```python
from build123d import *

# Parameters (mm, degrees)
IZIM1_R                     = 16
Y_KSEKLIK_EKSTR_ZYON1_DEPTH = 5
IZIM2_R                     = 8
Y_KSEKLIK_EKSTR_ZYON2_DEPTH = 19.7
KES_EKSTR_ZYON1_REACH       = 35.498
IZIM3_R                     = 4
KES_EKSTR_ZYON2_REACH       = 35.498
IZIM4_R                     = 1.75
IZIM4_3_R                   = 3.25
IZIM4_3_R_2                 = 1.75
KES_EKSTR_ZYON3_DEPTH       = 3.7
IZIM5_R                     = 6.5
KES_EKSTR_ZYON4_DEPTH       = 1.3
KES_EKSTR_ZYON5_START       = -23.4
IZIM5_2_R                   = 6.5
KES_EKSTR_ZYON5_DEPTH       = 1.3
KES_EKSTR_ZYON7_START       = -0.3
IZIM7_R                     = 9.5
IZIM7_R_2                   = 8
KES_EKSTR_ZYON7_DEPTH       = 0.3
IZIM8_R                     = 8
IZIM8_R_2                   = 7.5
KES_EKSTR_ZYON8_DEPTH       = 1
PAH1_SIZE                   = 0.5
Y_KSEKLIK_EKSTR_ZYON3_START = 0.5
IZIM9_R                     = 4.5
IZIM9_R_2                   = 4
Y_KSEKLIK_EKSTR_ZYON3_DEPTH = 0.5
Y_KSEKLIK_EKSTR_ZYON4_START = -22.1
IZIM9_2_R                   = 4.5
IZIM9_2_R_2                 = 4
Y_KSEKLIK_EKSTR_ZYON4_DEPTH = 0.5
PAH2_SIZE                   = 0.5


with BuildPart() as part:
    # Çizim1 → Yükseklik-Ekstrüzyon1 (new body)
    with BuildSketch(Plane.XY):
        Circle(IZIM1_R)
    extrude(amount=Y_KSEKLIK_EKSTR_ZYON1_DEPTH)

    # Çizim2 → Yükseklik-Ekstrüzyon2 (add)
    with BuildSketch(Plane.XY.offset(5)):
        Circle(IZIM2_R)
    extrude(amount=Y_KSEKLIK_EKSTR_ZYON2_DEPTH)

    # Çizim3 → Kes-Ekstrüzyon1 (cut, up to next)
    with BuildSketch(Plane.XY.offset(24.7), mode=Mode.PRIVATE) as kes_ekstr_zyon1_sk1:
        Circle(IZIM3_R)
    kes_ekstr_zyon1_tool1 = extrude(kes_ekstr_zyon1_sk1.sketch, amount=-KES_EKSTR_ZYON1_REACH, mode=Mode.PRIVATE) & part.part
    add(kes_ekstr_zyon1_tool1.solids().sort_by_distance((0, 0, 24.7))[0], mode=Mode.SUBTRACT)

    # Çizim4 → Kes-Ekstrüzyon2 (cut, up to next)
    with BuildSketch(Plane(origin=(0, 0, 0), x_dir=(-1, 0, 0), z_dir=(0, 0, -1)), mode=Mode.PRIVATE) as kes_ekstr_zyon2_sk1:
        with Locations((0, 12)):
            Circle(IZIM4_R)
    kes_ekstr_zyon2_tool1 = extrude(kes_ekstr_zyon2_sk1.sketch, amount=-KES_EKSTR_ZYON2_REACH, mode=Mode.PRIVATE) & part.part
    # Çizim4 → Kes-Ekstrüzyon2 (cut, up to next)
    with BuildSketch(Plane(origin=(0, 0, 0), x_dir=(-1, 0, 0), z_dir=(0, 0, -1)), mode=Mode.PRIVATE) as kes_ekstr_zyon2_sk2:
        with Locations((12, 0)):
            Circle(IZIM4_R)
    kes_ekstr_zyon2_tool2 = extrude(kes_ekstr_zyon2_sk2.sketch, amount=-KES_EKSTR_ZYON2_REACH, mode=Mode.PRIVATE) & part.part
    # Çizim4 → Kes-Ekstrüzyon2 (cut, up to next)
    with BuildSketch(Plane(origin=(0, 0, 0), x_dir=(-1, 0, 0), z_dir=(0, 0, -1)), mode=Mode.PRIVATE) as kes_ekstr_zyon2_sk3:
        with Locations((0, -12)):
            Circle(IZIM4_R)
    kes_ekstr_zyon2_tool3 = extrude(kes_ekstr_zyon2_sk3.sketch, amount=-KES_EKSTR_ZYON2_REACH, mode=Mode.PRIVATE) & part.part
    # Çizim4 → Kes-Ekstrüzyon2 (cut, up to next)
    with BuildSketch(Plane(origin=(0, 0, 0), x_dir=(-1, 0, 0), z_dir=(0, 0, -1)), mode=Mode.PRIVATE) as kes_ekstr_zyon2_sk4:
        with Locations((-12, 0)):
            Circle(IZIM4_R)
    kes_ekstr_zyon2_tool4 = extrude(kes_ekstr_zyon2_sk4.sketch, amount=-KES_EKSTR_ZYON2_REACH, mode=Mode.PRIVATE) & part.part
    add(kes_ekstr_zyon2_tool1.solids().sort_by_distance((0, 12, 0))[0], mode=Mode.SUBTRACT)
    add(kes_ekstr_zyon2_tool2.solids().sort_by_distance((-12, 0, 0))[0], mode=Mode.SUBTRACT)
    add(kes_ekstr_zyon2_tool3.solids().sort_by_distance((0, -12, 0))[0], mode=Mode.SUBTRACT)
    add(kes_ekstr_zyon2_tool4.solids().sort_by_distance((12, 0, 0))[0], mode=Mode.SUBTRACT)

    # Çizim4<3> → Kes-Ekstrüzyon3 (cut)
    # profile 1 of 4: a face of its own
    with BuildSketch(Plane(origin=(0, 0, 0), x_dir=(-1, 0, 0), z_dir=(0, 0, -1))):
        with Locations((0, 12)):
            Circle(IZIM4_3_R)
        with Locations((0, 12)):
            Circle(IZIM4_3_R_2, mode=Mode.SUBTRACT)
    # profile 2 of 4: a face of its own
    with BuildSketch(Plane(origin=(0, 0, 0), x_dir=(-1, 0, 0), z_dir=(0, 0, -1))):
        with Locations((12, 0)):
            Circle(IZIM4_3_R)
        with Locations((12, 0)):
            Circle(IZIM4_3_R_2, mode=Mode.SUBTRACT)
    # profile 3 of 4: a face of its own
    with BuildSketch(Plane(origin=(0, 0, 0), x_dir=(-1, 0, 0), z_dir=(0, 0, -1))):
        with Locations((0, -12)):
            Circle(IZIM4_3_R)
        with Locations((0, -12)):
            Circle(IZIM4_3_R_2, mode=Mode.SUBTRACT)
    # profile 4 of 4: a face of its own
    with BuildSketch(Plane(origin=(0, 0, 0), x_dir=(-1, 0, 0), z_dir=(0, 0, -1))):
        with Locations((-12, 0)):
            Circle(IZIM4_3_R)
        with Locations((-12, 0)):
            Circle(IZIM4_3_R_2, mode=Mode.SUBTRACT)
    extrude(amount=-KES_EKSTR_ZYON3_DEPTH, mode=Mode.SUBTRACT)

    # Çizim5 → Kes-Ekstrüzyon4 (cut)
    with BuildSketch(Plane.XY.offset(24.7)):
        Circle(IZIM5_R)
    extrude(amount=-KES_EKSTR_ZYON4_DEPTH, mode=Mode.SUBTRACT)

    # Çizim5<2> → Kes-Ekstrüzyon5 (cut)
    with BuildSketch(Plane.XY.offset(24.7).offset(KES_EKSTR_ZYON5_START)):
        Circle(IZIM5_2_R)
    extrude(amount=-KES_EKSTR_ZYON5_DEPTH, mode=Mode.SUBTRACT)

    # Çizim7 → Kes-Ekstrüzyon7 (cut)
    with BuildSketch(Plane.XY.offset(5).offset(KES_EKSTR_ZYON7_START)):
        Circle(IZIM7_R)
        Circle(IZIM7_R_2, mode=Mode.SUBTRACT)
    extrude(amount=KES_EKSTR_ZYON7_DEPTH, mode=Mode.SUBTRACT)

    # Çizim8 → Kes-Ekstrüzyon8 (cut)
    with BuildSketch(Plane.XY.offset(4.7)):
        Circle(IZIM8_R)
        Circle(IZIM8_R_2, mode=Mode.SUBTRACT)
    extrude(amount=KES_EKSTR_ZYON8_DEPTH, mode=Mode.SUBTRACT)

    # Pah1
    pah1_edges = [part.edges().sort_by_distance(p)[0] for p in [
        (-7.5, 0, 5.7),
    ]]
    chamfer(pah1_edges, length=PAH1_SIZE - 0.0001)  # a hair under: the kernel refuses the full size

    # Çizim9 → Yükseklik-Ekstrüzyon3 (add)
    with BuildSketch(Plane.XY.offset(23.4).offset(Y_KSEKLIK_EKSTR_ZYON3_START)):
        Circle(IZIM9_R)
        Circle(IZIM9_R_2, mode=Mode.SUBTRACT)
    extrude(amount=-Y_KSEKLIK_EKSTR_ZYON3_DEPTH)

    # Çizim9<2> → Yükseklik-Ekstrüzyon4 (add)
    with BuildSketch(Plane.XY.offset(23.4).offset(Y_KSEKLIK_EKSTR_ZYON4_START)):
        Circle(IZIM9_2_R)
        Circle(IZIM9_2_R_2, mode=Mode.SUBTRACT)
    extrude(amount=-Y_KSEKLIK_EKSTR_ZYON4_DEPTH)

    # Pah2
    pah2_edges = [part.edges().sort_by_distance(p)[0] for p in [
        (-16, 0, 0),
        (-16, 0, 5),
        (-8, 0, 24.7),
    ]]
    chamfer(pah2_edges, length=PAH2_SIZE)


solid = part.part
```
Geometry check sheet. Reference: the model listing, model coordinates, mm. A direction names the side the tool comes from. Round coordinates to 2 decimals unless told otherwise and drop trailing zeros. Loops run counter-clockwise (first coordinate to the right, second up) from the corner with the lowest first, then second, coordinate; pieces in that order, holes last. Notation, with made-up numbers: (52, 51) - (107, 51) arc R17 ccw to (107, 80) - close; hole circle Ø1 at (26.25, -35.75). An arc over 180 degrees is marked (long way). Write item = value, one per line. Start each with the question number.
1. Depth check by flat-ended pin: pin 1 (10.5 mm diameter, centred on x = 0, y = 0, fed in from +Z); pin 2 (10 mm diameter, centred on y = 10, z = 14, fed in from -X) (3 decimals); pin 3 (5 mm diameter, centred on x = -12, y = 0, fed in from +Z). Enter the tip coordinate at first touch or a pass-through.
2. Mould release check, pull along X, two halves, no side actions. Record for faces 4 (the face through (-3.47, -15.62, 2.47)), 5 (the face through (7, 7, 5)), 6 (the face through (0.228, -10.265, 4.341)): released by +X, released by -X, zero draft, split by the parting line, or undercut.
3. Thickness scan on line 1 (Y direction, x = 0, z = 17.5); line 2 (Y direction, x = 0, z = 4.6); line 3 (Y direction, x = 0, z = 1.75). Record the ranges inside material, lowest first.
4. Section check A-A on y = 0. Give the number of separate pieces and of enclosed holes in the cut face, then the cut area to 3 significant figures.
5. Section check C-C on z = 13.75. Enter the section's corners in (x, y).
6. Set-up check for faces 1 (the face through (-5.158, -3.955, 24.059)), 2 (the face through (1, 8, 4.7)), 3 (the face through (-5.158, -3.955, 0.659)): record each of +Z, -Z, +X, -X, +Y, -Y from which the full face is reachable in a straight line by a thin tool's end or side.
Working result:
q1.pin_1 = 23.9
q1.pin_2 = -6.245
q1.pin_3 = 5
q2.face_4 = split by the parting line
q2.face_5 = zero draft
q2.face_6 = undercut
q3.line_1 = -8 to -4, 4 to 8
q3.line_2 = -15.9 to -13.75, -10.25 to -4, 4 to 10.25, 13.75 to 15.9
q3.line_3 = -16 to -15.25, -8.75 to -4, 4 to 8.75, 15.25 to 16
q4.separate_pieces = 4
q4.enclosed_holes = 0
q4.area = 206 mm^2
q5.outline = circle Ø16 at (0, 0); hole circle Ø8 at (0, 0)
q6.face_1 = +Z
q6.face_2 = none
q6.face_3 = -Z
